The model under review builds one solid part; all positions refer to its coordinate system, in mm. A direction names the side the tool comes from. Round coordinates to 2 decimals unless told otherwise and drop trailing zeros. Write each loop counter-clockwise with the first axis right and the second up, starting at its lowest first coordinate (ties: lowest second). Pieces come first, ordered by that corner, then holes. Notation, with made-up numbers: (-13.5, 31.5) -> (6.5, 31.5) arc R7 ccw to (6.5, 38.5) -> close; hole circle Ø10 at (60.5, 45.5). An arc over 180 degrees is marked (long way). Answer as a JSON object with one key per item and string values. Group by question number.
1) We need section C-C, the plane y = 55. Write out the cut boundary in (x, z).
2) Mouldability with a two-part tool opening along Y and no side actions: class faces 1 (the flat face through (-2, 50, 7)), 2 (the flat face through (-2, -75, 6)), 3 (the flat face through (175, -1, 6)), 4 (the flat face through (-2, 75, 6)) as pulls with the +Y half, pulls with the -Y half, needs draft (parallel to the pull), parting line crosses it, or undercut.
3) To check wall thickness, follow probe 1 along Y at (x, z) = (2, 11.5); probe 2 along Y at (x, z) = (53.5, 6.75); probe 3 along X at (y, z) = (22.5, 5.5). State the ranges of each line that lie inside material, in increasing order. Write a range as [from, to].
4) We need section B-B, the plane x = -6.5. Write out the cut boundary in (y, z), then the cut area to 3 significant figures.
5) We need section A-A, the plane z = 9.25. Write out the cut boundary in (x, y).
6) Insertion check: pin 1 Ø3 at (x, y) = (-40.5, 22) entering from +Z. The pin has a flat end and moves straight along its axis. Give the tip position at first contact, or say it passes through.
7) Machinability: for faces 5 (the flat face through (-71, 28.269, 7)), 6 (the flat face through (-175, -1, 6)), which of the approach directions +Z, -Z, +X, -X, +Y, -Y give a long, thin tool a straight path to every point of the face, cutting with its end or side? Answer none if there is none.
from build123d import *

# Parameters (mm, degrees)
F0_W     = 350
F0_H     = 150
F1_DEPTH = 12
F3_DEPTH = 10


with BuildPart() as f1:
    # F0 (on Top) → F1 (new body)
    with BuildSketch(Plane.XY):
        Rectangle(F0_W, F0_H)
    extrude(amount=F1_DEPTH)

    # F2 (on face) → F3 (cut)
    with BuildSketch(Plane.XY.offset(12)):
        with BuildLine():
            Line((148, 60), (-148, 60))
            ThreePointArc((-148, 60), (-153, 55), (-148, 50))
            Line((-148, 50), (148, 50))
            ThreePointArc((148, 50), (153, 55), (148, 60))
        make_face()
        with BuildLine():
            ThreePointArc((2.280964, 18.268998), (7.280964, 23.268998), (2.280964, 28.268998))
            Line((2.280964, 28.268998), (-146.719036, 28.268998))
            ThreePointArc((-146.719036, 28.268998), (-151.719036, 23.268998), (-146.719036, 18.268998))
            Line((-146.719036, 18.268998), (2.280964, 18.268998))
        make_face()
    extrude(amount=-F3_DEPTH, mode=Mode.SUBTRACT)


solid = f1.part
Here are the results:
{
 "1": {"outline": "(-175, 0) -> (175, 0) -> (175, 12) -> (153, 12) -> (153, 2) -> (-153, 2) -> (-153, 12) -> (-175, 12) -> close"},
 "2": {"face 1": "undercut", "face 2": "pulls with the -Y half", "face 3": "needs draft", "face 4": "pulls with the +Y half"},
 "3": {"probe 1": "y = [-75, 18.27], [28.27, 50], [60, 75]", "probe 2": "y = [-75, 50], [60, 75]", "probe 3": "x = [-175, -151.66], [7.22, 175]"},
 "4": {"outline": "(-75, 0) -> (75, 0) -> (75, 12) -> (60, 12) -> (60, 2) -> (50, 2) -> (50, 12) -> (28.27, 12) -> (28.27, 2) -> (18.27, 2) -> (18.27, 12) -> (-75, 12) -> close", "area": "1,600 mm^2"},
 "5": {"outline": "(-175, -75) -> (175, -75) -> (175, 75) -> (-175, 75) -> close; hole (-148, 50) -> (148, 50) arc R5 ccw to (148, 60) -> (-148, 60) arc R5 ccw to start; hole (-146.72, 18.27) -> (2.28, 18.27) arc R5 ccw to (2.28, 28.27) -> (-146.72, 28.27) arc R5 ccw to start"},
 "6": {"pin 1": "stops at z = 2"},
 "7": {"face 5": "+Z", "face 6": "+Z, -Z, -X, +Y, -Y"}
}
